Verification items for the finished model (mm, model axes). Round coordinates to 2 decimals unless told otherwise and drop trailing zeros. Write each loop counter-clockwise with the first axis right and the second up, starting at its lowest first coordinate (ties: lowest second). Pieces come first, ordered by that corner, then holes. Notation, with made-up numbers: M 21.25,36 L 48.25,36 A21 ccw 48.25,49 Z; hole C 64.25,45 d6. An arc over 180 degrees is marked long. One line per question, with ' | ' between items. Start each with the question number.
Q1. Cross-section at A-A (y = -2.5). Record the boundary of the cut face in (x, z), then the cut area to 3 significant figures.
Q2. Thickness scan on line 1 along Z through (x, y) = (194, -0.8); line 2 along X through (y, z) = (-3.65, 865.5); line 3 along Z through (x, y) = (235, -0.65). Record the ranges inside material, lowest first. Write a range as from..to.
Q3. Gauge pin test, flat end, axial feed: pin 1 (2 mm diameter, centred on x = 409.5, y = -2.5, fed in from +Z). Record the tip position at first contact, or that the pin passes through.
from build123d import *

# Parameters (mm, degrees)
F1_DEPTH = 4
F2_SIZE  = 3.99999
F4_DEPTH = 25


# Not quite as in the source:
# - a fillet or chamfer is up to 0.001 mm smaller than in the source, because OpenCascade refuses the exact size
# - ends of sketch curves that miss each other by under 0.0002 mm in the source are joined


with BuildPart() as f1:
    # F0 (on Front) → F1 (new body)
    with BuildSketch(Plane.XZ):
        Polygon((0, 944.56), (0, 0), (412.03, 0), (412.03, 532.53), align=None)
    extrude(amount=F1_DEPTH)

    # F2 (size 4 in the source; OpenCascade refuses exactly that, so slightly less here)
    f2_edges = [f1.edges().sort_by_distance(p)[0] for p in [
        (206.015, 0, 738.545),
    ]]
    chamfer(f2_edges, length=F2_SIZE)

    # F3 (on face) → F4 (join)
    with BuildSketch(Plane.YZ.offset(412.03)):
        Polygon((-3.99999, 532.53), (0, 526.8731598926), (0, 532.53), align=None)
    extrude(amount=-F4_DEPTH)


solid = f1.part
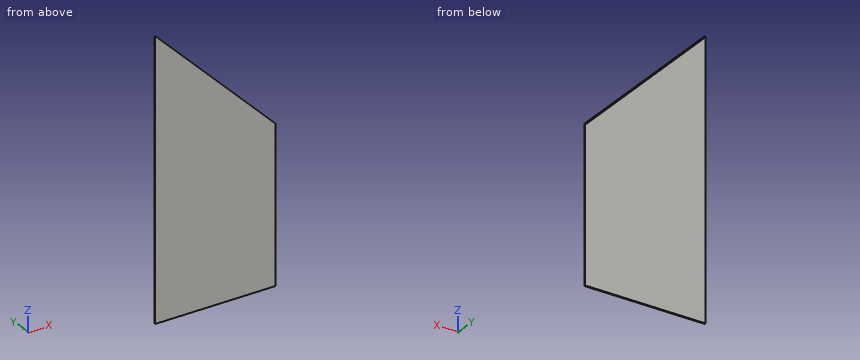
Determined:
1) outline: M 0,0 L 412.03,0 L 412.03,532.53 L 409.91,532.53 L 0,942.44 Z | area: 303,000 mm²
2) line 1: z = 0..746.03 | line 2: x = 0..78.57 | line 3: z = 0..704.82
3) pin 1: stops at z = 534.67
